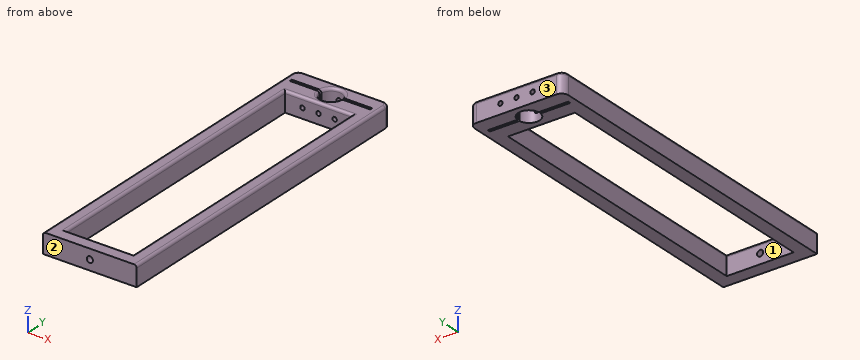
from build123d import *

# Parameters (mm, degrees)
SKETCH_1_W          = 70
SKETCH_1_H          = 15
EXTRUDE_3_DEPTH     = 254
SKETCH_5_W          = 50
SKETCH_5_H          = 219
CUT_EXTRUDE_2_DEPTH = 150
SKETCH_6_R          = 8
CUT_EXTRUDE_3_DEPTH = 150
FILLET_1_R          = 2
FILLET_2_R          = 5
FILLET_3_R          = 5
SKETCH_7_R          = 2.3
CUT_EXTRUDE_4_DEPTH = 150
SKETCH_8_W          = 60
SKETCH_8_H          = 2
CUT_EXTRUDE_5_DEPTH = 257.838470639
FILLET_4_R          = 2
FILLET_7_R          = 2
SKETCH_9_R          = 1.65
CUT_EXTRUDE_6_DEPTH = 30


with BuildPart() as part:
    # 草图1 → 凸台-拉伸3 (new body)
    with BuildSketch(Plane(origin=(0, 0, 0), x_dir=(1, 0, 0), z_dir=(0, 1, 0))):
        Rectangle(SKETCH_1_W, SKETCH_1_H)
    extrude(amount=EXTRUDE_3_DEPTH)

    # 草图5 → 切除-拉伸2 (cut)
    with BuildSketch(Plane.XY.offset(7.5)):
        with Locations((0, 119.5)):
            Rectangle(SKETCH_5_W, SKETCH_5_H)
    extrude(amount=-CUT_EXTRUDE_2_DEPTH, mode=Mode.SUBTRACT)

    # 草图6 → 切除-拉伸3 (cut)
    with BuildSketch(Plane.XY.offset(7.5)):
        with Locations((0, 241.5)):
            Circle(SKETCH_6_R)
    extrude(amount=-CUT_EXTRUDE_3_DEPTH, mode=Mode.SUBTRACT)

    # 圆角1
    fillet_1_edges = [part.edges().sort_by_distance(p)[0] for p in [
        (-8, 241.5, 7.5),
    ]]
    fillet(fillet_1_edges, radius=FILLET_1_R)

    # 圆角2
    fillet_2_edges = [part.edges().sort_by_distance(p)[0] for p in [
        (-35, 254, 0),
    ]]
    fillet(fillet_2_edges, radius=FILLET_2_R)

    # 圆角3
    fillet_3_edges = [part.edges().sort_by_distance(p)[0] for p in [
        (35, 254, 0),
    ]]
    fillet(fillet_3_edges, radius=FILLET_3_R)

    # 草图7 → 切除-拉伸4 (cut)
    with BuildSketch(Plane(origin=(0, 10, 0), x_dir=(1, 0, 0), z_dir=(0, 1, 0))):
        with Locations(Location((0, 0, 0), (0, 0, 270))):
            Circle(SKETCH_7_R)
    extrude(amount=-CUT_EXTRUDE_4_DEPTH, mode=Mode.SUBTRACT)

    # 草图8 → 切除-拉伸5 (cut, through all)
    with BuildSketch(Plane(origin=(0, 0, -7.5), x_dir=(-1, 0, 0), z_dir=(0, 0, -1))):
        with Locations((0, 241.5)):
            Rectangle(SKETCH_8_W, SKETCH_8_H)
    extrude(amount=-CUT_EXTRUDE_5_DEPTH, mode=Mode.SUBTRACT)

    # 圆角4
    fillet_4_edges = [part.edges().sort_by_distance(p)[0] for p in [
        (-35, 124.5, 7.5),
        (0, 254, 7.5),
        (-33.535533906, 252.535533906, 7.5),
        (35, 124.5, 7.5),
        (33.535533906, 252.535533906, 7.5),
    ]]
    fillet(fillet_4_edges, radius=FILLET_4_R)

    # 圆角7
    fillet_7_edges = [part.edges().sort_by_distance(p)[0] for p in [
        (-25, 119.5, 7.5),
        (0, 10, 7.5),
        (25, 119.5, 7.5),
        (0, 229, 7.5),
    ]]
    fillet(fillet_7_edges, radius=FILLET_7_R)

    # 草图9 → 切除-拉伸6 (cut)
    with BuildSketch(Plane(origin=(0, 254, 0), x_dir=(1, 0, 0), z_dir=(0, 1, 0))):
        with Locations(Location((-12, 0, 0), (0, 0, 270))):
            Circle(SKETCH_9_R)
        with Locations(Location((12, 0, 0), (0, 0, 270))):
            Circle(SKETCH_9_R)
        with Locations(Location((0, 0, 0), (0, 0, 270))):
            Circle(SKETCH_9_R)
    extrude(amount=-CUT_EXTRUDE_6_DEPTH, mode=Mode.SUBTRACT)


solid = part.part
Source: CAD feature listing. Evaluate the final solid. Frame: model axes, mm. Face numbers are marked on the shaded views. Round coordinates to 2 decimals unless told otherwise and drop trailing zeros. Write each loop counter-clockwise with the first axis right and the second up, starting at its lowest first coordinate (ties: lowest second). Pieces come first, ordered by that corner, then holes. Notation, with made-up numbers: M 64.25,37.25 L 103.25,37.25 A19 cw 103.25,54.25 Z; hole C 20,8.5 d7. An arc over 180 degrees is marked long. One line per item, written item: value. Start each with the question number.
Item 1: Mould query, pull axis Y, two halves, no side actions, for the marked faces 1, 2 and 3. Classes: pulls with the +Y half, pulls with the -Y half, needs draft (parallel to the pull), parting line crosses it, or undercut.
Item 2: Ray query, L1, parallel to Y at x = 1.5, z = -6; L2, parallel to X at y = 232.25, z = 0; L3, parallel to Y at x = 8, z = 5.75. Return the intervals inside material, ascending. Write a range as from..to.
Item 3: Pin query (flat end, axial travel): pin 1 (2.5 mm diameter, centred on x = -12, z = 0, fed in from +Y). Return the tip coordinate at first contact, or that it passes through.
Item 4: Section query A-A (y = 121). Return the cut outline in (x, z).
Result set:
1. face 1: undercut
1. face 2: pulls with the -Y half
1. face 3: pulls with the +Y half
2. L1: y = 0..10, 229..233.64, 249.36..254
2. L2: x = -35..-13.65, -10.35..-1.65, 1.65..10.35, 13.65..35
2. L3: y = 0..9.98, 229.02..240.5, 242.5..253.98
3. pin 1: stops at y = 10
4. outline: M -35,-7.5 L -25,-7.5 L -25,5.5 A2 ccw -27,7.5 L -33,7.5 A2 ccw -35,5.5 Z; M 25,-7.5 L 35,-7.5 L 35,5.5 A2 ccw 33,7.5 L 27,7.5 A2 ccw 25,5.5 Z
